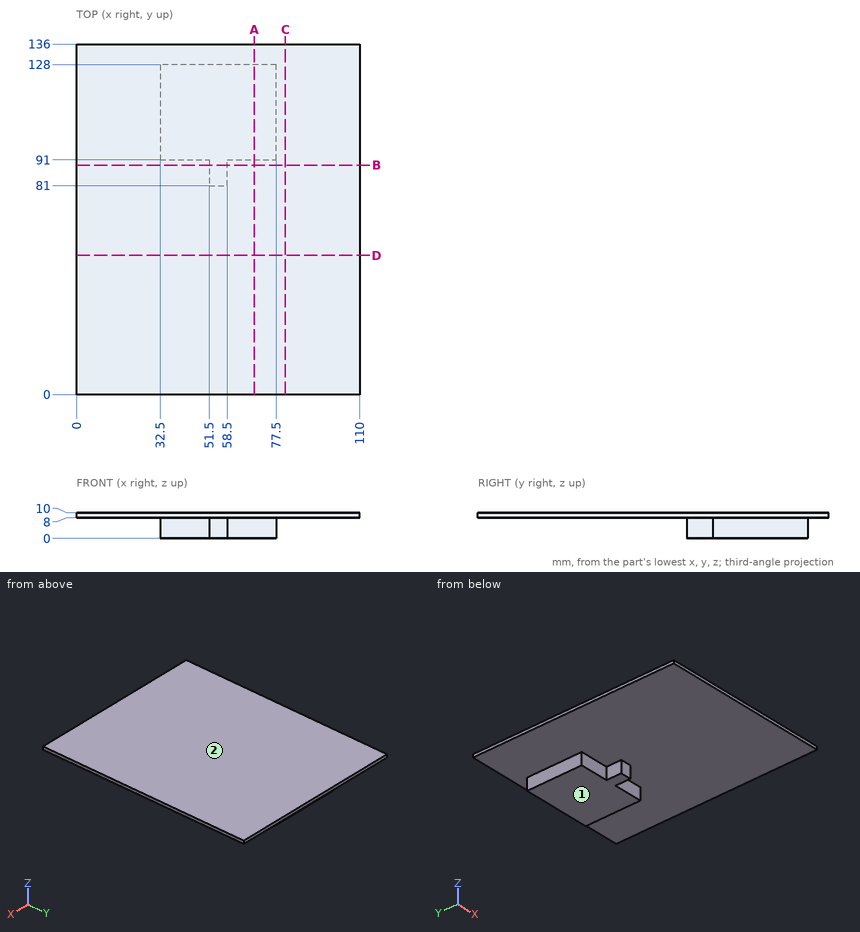
Check sheet for the drawn part. Datum: minimum x, y, z corner. Units: mm. Coordinates: 2 decimals unless noted, no trailing zeros. Write each loop counter-clockwise with the first axis right and the second up, starting at its lowest first coordinate (ties: lowest second). Pieces come first, ordered by that corner, then holes. Notation, with made-up numbers: M -27,23.25 L -1,23.25 A19 ccw -1,40.25 Z; hole C 6.5,17 d4. An arc over 180 degrees is marked long. One line per item, written item: value.
Item 1: Section check C-C, the plane x = 81. Record the boundary of the cut face in (y, z), plus the area to 3 significant figures.
Check sheet entries:
outline: M 0,8 L 136,8 L 136,10 L 0,10 Z
area: 272 mm^2
Item 2: Gauge pin test, flat ends, axial feed: pin 1 Ø2.5 at (y, z) = (86.5, 5) entering from -X; pin 2 Ø4 at (x, z) = (67, 2.5) entering from -Y; pin 3 Ø12 at (x, y) = (24.5, 82.5) entering from -Z. Record the tip position at first contact, or that the pin passes through.
Check sheet entries:
pin 1: stops at x = 51.5
pin 2: stops at y = 91
pin 3: stops at z = 8
Item 3: Section check D-D, the plane y = 54. Record the boundary of the cut face in (x, z).
Check sheet entries:
outline: M 0,8 L 110,8 L 110,10 L 0,10 Z
Item 4: Section check A-A, the plane x = 69. Record the boundary of the cut face in (y, z).
Check sheet entries:
outline: M 0,8 L 91,8 L 91,0 L 128,0 L 128,8 L 136,8 L 136,10 L 0,10 Z
Item 5: Mould release check, pull along Z, two halves, no side actions. Record for the marked faces 1 and 2: pulls with the +Z half, pulls with the -Z half, needs draft (parallel to the pull), parting line crosses it, or undercut.
Check sheet entries:
face 1: pulls with the -Z half
face 2: pulls with the +Z half
Item 6: Scan lines: line 1 along Z through (x, y) = (29, 67.5); line 2 along Y through (x, z) = (71, 2.75); line 3 along Y through (x, z) = (57, 3). Record each from-to range of solid material in increasing order.
Check sheet entries:
line 1: z = 8 to 10
line 2: y = 91 to 128
line 3: y = 81 to 128
Item 7: Section check B-B, the plane y = 89. Record the boundary of the cut face in (x, z), plus the area to 3 significant figures.
Check sheet entries:
outline: M 0,8 L 51.5,8 L 51.5,0 L 58.5,0 L 58.5,8 L 110,8 L 110,10 L 0,10 Z
area: 276 mm^2
